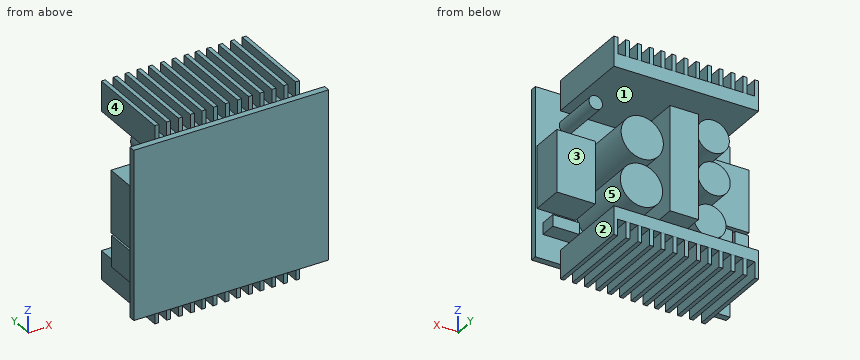
from build123d import *

# Parameters (mm, degrees)
SKIZZE1_W                        = 60
SKIZZE1_H                        = 52
AUFSATZ_LINEAR_AUSTRAGEN1_DEPTH  = 2
SKIZZE2_W                        = 4.171328817
SKIZZE2_H                        = 9.629375294
SKIZZE2_H_2                      = 9.629375295
AUFSATZ_LINEAR_AUSTRAGEN2_DEPTH  = 10
SKIZZE3_W                        = 11.843772269
SKIZZE3_H                        = 19.121604294
SKIZZE3_H_2                      = 19.121604293
AUFSATZ_LINEAR_AUSTRAGEN3_DEPTH  = 10
SKIZZE4_R                        = 2.072288809
AUFSATZ_LINEAR_AUSTRAGEN4_DEPTH  = 15
SKIZZE5_W                        = 8.191020073
SKIZZE5_H                        = 3.542062735
AUFSATZ_LINEAR_AUSTRAGEN5_DEPTH  = 5
SKIZZE6_W                        = 44.607852562
SKIZZE6_H                        = 3.763441655
SKIZZE6_H_2                      = 4.206199497
AUFSATZ_LINEAR_AUSTRAGEN6_DEPTH  = 27
SKIZZE7_R                        = 5
SKIZZE7_R_2                      = 6.5
AUFSATZ_LINEAR_AUSTRAGEN7_DEPTH  = 22
SKIZZE8_W                        = 8.773032398
SKIZZE8_H                        = 32.167785459
AUFSATZ_LINEAR_AUSTRAGEN8_DEPTH  = 25
SKIZZE9_W                        = 1.22
SKIZZE9_H                        = 27
SKIZZE9_W_2                      = 1.198395349
SKIZZE9_H_2                      = 26.967916188
SKIZZE9_W_3                      = 1.238034023
AUFSATZ_LINEAR_AUSTRAGEN9_DEPTH  = 5
SKIZZE10_W                       = 1.22
SKIZZE10_H                       = 27
SKIZZE10_W_2                     = 1.198395349
SKIZZE10_H_2                     = 26.967916188
SKIZZE10_W_3                     = 1.196647202
AUFSATZ_LINEAR_AUSTRAGEN10_DEPTH = 5


with BuildPart() as part:
    # Skizze1 → Aufsatz-Linear austragen1 (new body)
    with BuildSketch(Plane(origin=(0, 0, 0), x_dir=(1, 0, 0), z_dir=(0, 1, 0))):
        Rectangle(SKIZZE1_W, SKIZZE1_H)
    extrude(amount=AUFSATZ_LINEAR_AUSTRAGEN1_DEPTH)

    # Skizze2 → Aufsatz-Linear austragen2 (add)
    with BuildSketch(Plane(origin=(0, 2, 0), x_dir=(1, 0, 0), z_dir=(0, 1, 0))):
        with Locations((-27.429980224, 11.040969798)):
            Rectangle(SKIZZE2_W, SKIZZE2_H)
        with Locations((-22.466389845, 11.024313198)):
            Rectangle(SKIZZE2_W, SKIZZE2_H_2)
    extrude(amount=AUFSATZ_LINEAR_AUSTRAGEN2_DEPTH)

    # Skizze3 → Aufsatz-Linear austragen3 (add)
    with BuildSketch(Plane(origin=(0, 2, 0), x_dir=(1, 0, 0), z_dir=(0, 1, 0))):
        with Locations((23.554785505, 1.549851865)):
            Rectangle(SKIZZE3_W, SKIZZE3_H)
        with Locations((-23.759716727, -4.226654643)):
            Rectangle(SKIZZE3_W, SKIZZE3_H_2)
    extrude(amount=AUFSATZ_LINEAR_AUSTRAGEN3_DEPTH)

    # Skizze4 → Aufsatz-Linear austragen4 (add)
    with BuildSketch(Plane(origin=(0, 2, 0), x_dir=(1, 0, 0), z_dir=(0, 1, 0))):
        with Locations(Location((20.536465542, -16.425780337, 0), (0, 0, 90))):
            Circle(SKIZZE4_R)
    extrude(amount=AUFSATZ_LINEAR_AUSTRAGEN4_DEPTH)

    # Skizze5 → Aufsatz-Linear austragen5 (add)
    with BuildSketch(Plane(origin=(0, 2, 0), x_dir=(1, 0, 0), z_dir=(0, 1, 0))):
        with Locations((23.538626636, 16.697381153)):
            Rectangle(SKIZZE5_W, SKIZZE5_H)
    extrude(amount=AUFSATZ_LINEAR_AUSTRAGEN5_DEPTH)

    # Skizze6 → Aufsatz-Linear austragen6 (add)
    with BuildSketch(Plane(origin=(0, 2, 0), x_dir=(1, 0, 0), z_dir=(0, 1, 0))):
        with Locations((0, 23.549182712)):
            Rectangle(SKIZZE6_W, SKIZZE6_H)
        with Locations((0, -23.05108014)):
            Rectangle(SKIZZE6_W, SKIZZE6_H_2)
    extrude(amount=AUFSATZ_LINEAR_AUSTRAGEN6_DEPTH)

    # Skizze7 → Aufsatz-Linear austragen7 (add)
    with BuildSketch(Plane(origin=(0, 2, 0), x_dir=(1, 0, 0), z_dir=(0, 1, 0))):
        with Locations(Location((-11.604540209, 0.487390689, 0), (0, 0, 90))):
            Circle(SKIZZE7_R)
        with Locations(Location((-10.304831705, 13.855821009, 0), (0, 0, 90))):
            Circle(SKIZZE7_R)
        with Locations(Location((-11.326031244, -12.324021702, 0), (0, 0, 90))):
            Circle(SKIZZE7_R)
        with Locations(Location((10.722595153, 9.353259408, 0), (0, 0, 90))):
            Circle(SKIZZE7_R_2)
        with Locations(Location((10.490504349, -5.268461255, 0), (0, 0, 90))):
            Circle(SKIZZE7_R_2)
    extrude(amount=AUFSATZ_LINEAR_AUSTRAGEN7_DEPTH)

    # Skizze8 → Aufsatz-Linear austragen8 (add)
    with BuildSketch(Plane(origin=(0, 2, 0), x_dir=(1, 0, 0), z_dir=(0, 1, 0))):
        with Locations((-0.626645171, 0.417763447)):
            Rectangle(SKIZZE8_W, SKIZZE8_H)
    extrude(amount=AUFSATZ_LINEAR_AUSTRAGEN8_DEPTH)

    # Skizze9 → Aufsatz-Linear austragen9 (add)
    with BuildSketch(Plane.XY.offset(25.154179888)):
        with Locations((-21.693926281, 15.5)):
            Rectangle(SKIZZE9_W, SKIZZE9_H)
        with Locations((-18.033926281, 15.513977132)):
            Rectangle(SKIZZE9_W, SKIZZE9_H)
        with Locations((-14.373926281, 15.548375388)):
            Rectangle(SKIZZE9_W, SKIZZE9_H)
        with Locations((-10.713926281, 15.56235252)):
            Rectangle(SKIZZE9_W, SKIZZE9_H)
        with Locations((-7.186859691, 15.565574516)):
            Rectangle(SKIZZE9_W, SKIZZE9_H)
        with Locations((-3.537662017, 15.563509742)):
            Rectangle(SKIZZE9_W_2, SKIZZE9_H_2)
        with Locations((0.050366666, 15.53117626)):
            Rectangle(SKIZZE9_W, SKIZZE9_H)
        with Locations((3.793140309, 15.462379749)):
            Rectangle(SKIZZE9_W, SKIZZE9_H)
        with Locations((10.692247294, 15.44141405)):
            Rectangle(SKIZZE9_W, SKIZZE9_H)
        with Locations((14.352247294, 15.455391183)):
            Rectangle(SKIZZE9_W, SKIZZE9_H)
        with Locations((18.012247294, 15.489789438)):
            Rectangle(SKIZZE9_W, SKIZZE9_H)
        with Locations((7.20130698, 15.513977132)):
            Rectangle(SKIZZE9_W, SKIZZE9_H)
        with Locations((21.68490927, 15.5)):
            Rectangle(SKIZZE9_W_3, SKIZZE9_H)
    extrude(amount=AUFSATZ_LINEAR_AUSTRAGEN9_DEPTH)

    # Skizze10 → Aufsatz-Linear austragen10 (add)
    with BuildSketch(Plane(origin=(0, 0, -25.430903539), x_dir=(-1, 0, 0), z_dir=(0, 0, -1))):
        with Locations((-18.033926281, 15.565538052)):
            Rectangle(SKIZZE10_W, SKIZZE10_H)
        with Locations((-14.373926281, 15.599936307)):
            Rectangle(SKIZZE10_W, SKIZZE10_H)
        with Locations((-10.713926281, 15.61391344)):
            Rectangle(SKIZZE10_W, SKIZZE10_H)
        with Locations((-7.186859691, 15.617135435)):
            Rectangle(SKIZZE10_W, SKIZZE10_H)
        with Locations((-3.537662017, 15.615070662)):
            Rectangle(SKIZZE10_W_2, SKIZZE10_H_2)
        with Locations((0.050366666, 15.58273718)):
            Rectangle(SKIZZE10_W, SKIZZE10_H)
        with Locations((3.793140309, 15.513940668)):
            Rectangle(SKIZZE10_W, SKIZZE10_H)
        with Locations((10.692247294, 15.49297497)):
            Rectangle(SKIZZE10_W, SKIZZE10_H)
        with Locations((14.352247294, 15.506952102)):
            Rectangle(SKIZZE10_W, SKIZZE10_H)
        with Locations((18.012247294, 15.541350358)):
            Rectangle(SKIZZE10_W, SKIZZE10_H)
        with Locations((7.20130698, 15.565538052)):
            Rectangle(SKIZZE10_W, SKIZZE10_H)
        with Locations((-21.70560268, 15.5)):
            Rectangle(SKIZZE10_W_3, SKIZZE10_H)
        with Locations((21.70560268, 15.5)):
            Rectangle(SKIZZE10_W_3, SKIZZE10_H)
    extrude(amount=AUFSATZ_LINEAR_AUSTRAGEN10_DEPTH)


solid = part.part
For this review, take the finished solid that the model builds, in its own axes (mm). Face numbers are marked on the shaded views. A direction names the side the tool comes from. Round coordinates to 2 decimals unless told otherwise and drop trailing zeros. Order: outer loops, then holes, each group sorted by start corner. A loop starts at its lowest first (then second) coordinate and runs counter-clockwise, first axis right, second up. Notation, with made-up numbers: M 47,36.5 L 83,36.5 A19 cw 83,47.5 Z; hole C 21.25,24.25 d5. An arc over 180 degrees is marked long. Use a Markdown table: item, result. Add a question column.
Item 1: Insertion check: pin 1 (2.5 mm diameter, centred on x = -1.5, y = 18.5, fed in from +Z); pin 2 (1.3 mm diameter, centred on x = -4, z = -28.5, fed in from +Y); pin 3 (1 mm diameter, centred on x = 20.5, y = 12, fed in from -Z); pin 4 (10.5 mm diameter, centred on x = 9.5, z = -6.5, fed in from +Y). Each pin has a flat end and moves straight along its axis. Give the tip position at first contact, or say it passes through.
Item 2: To check wall thickness, follow line 1 along Z through (x, y) = (0.5, 25.75); line 2 along X through (y, z) = (10.25, 12); line 3 along X through (y, z) = (15.5, 3). State the ranges of each line that lie inside material, in increasing order.
Item 3: Add section D-D, the plane z = -10. Give the boundary of the cut face in (x, y).
Item 4: Tool access review of the marked faces 1, 2 and 3: name each direction out of +Z, -Z, +X, -X, +Y, -Y from which nothing blocks a thin tool from reaching the whole face with its end or side.
Item 5: Add section B-B, the plane y = 21.5. State how many separate pieces and enclosed holes the cut face has, then the cut area to 3 significant figures.
Item 6: Mouldability with a two-part tool opening along Z and no side actions: class the marked faces 4 and 5 as released by +Z, released by -Z, zero draft, split by the parting line, or undercut.
Item 7: Add section A-A, the plane z = 5.5. Give the boundary of the cut face in (x, y), then the cut area to 3 significant figures.
Geometry results:
| question | item | result |
|---|---|---|
| 1 | pin 1 | stops at z = 30.15 |
| 1 | pin 2 | stops at y = 29.01 |
| 1 | pin 3 | stops at z = -25.43 |
| 1 | pin 4 | stops at y = 24 |
| 2 | line 1 | z = -30.43 to -21.67, -16.5 to 15.67, 20.95 to 30.15 |
| 2 | line 2 | x = -29.68 to -17.84, -16.32 to -6.34, -5.01 to 3.76 |
| 2 | line 3 | x = -15.19 to -8.02, -5.01 to 3.76, 4.4 to 16.58 |
| 3 | outline | M -30,0 L 30,0 L 30,2 L 29.48,2 L 29.48,12 L 17.63,12 L 17.63,2 L 17.19,2 L 17.19,24 L 4.25,24 L 4.25,2 L 3.76,2 L 3.76,27 L -5.01,27 L -5.01,2 L -7.12,2 L -7.12,24 L -13.49,24 L -13.49,2 L -20.38,2 L -20.38,12 L -24.55,12 L -24.55,2 L -25.34,2 L -25.34,12 L -29.52,12 L -29.52,2 L -30,2 Z |
| 4 | face 1 | +X, -X, +Y |
| 4 | face 2 | -Z, +X, +Y |
| 4 | face 3 | +X, +Y |
| 5 | separate pieces | 8 |
| 5 | enclosed holes | 0 |
| 5 | area | 1,300 mm² |
| 6 | face 4 | zero draft |
| 6 | face 5 | undercut |
| 7 | outline | M -30,0 L 30,0 L 30,2 L 29.48,2 L 29.48,12 L 17.63,12 L 17.63,2 L 16.99,2 L 16.99,24 L 3.99,24 L 3.99,2 L 3.76,2 L 3.76,27 L -5.01,27 L -5.01,2 L -17.84,2 L -17.84,12 L -29.68,12 L -29.68,2 L -30,2 Z |
| 7 | area | 862 mm² |
